Geometry check sheet. Reference: the model listing, model coordinates, mm. Give positions to 0.01 mm unless a question says otherwise; leave off trailing zeros. Order: outer loops, then holes, each group sorted by start corner. A loop starts at its lowest first (then second) coordinate and runs counter-clockwise, first axis right, second up. Notation, with made-up numbers: M 61.5,48.5 L 73.5,48.5 A10 cw 73.5,61.5 Z; hole C -32.5,-24.5 d10. An arc over 180 degrees is marked long. Answer as CSV lines item,"result". Start each with the question number.
Q1. Thickness scan on line 1 (Y direction, x = -12, z = -16.5); line 2 (Z direction, x = -14.25, y = 39.5); line 3 (Z direction, x = -20.25, y = 109). Record the ranges inside material, lowest first.
Q2. Go/stop test with flat-tipped pins: pin 1 (3.5 mm diameter, centred on x = -15.5, z = -15, fed in from -Y); pin 2 (2 mm diameter, centred on x = -14, y = 83, fed in from -Z); pin 3 (1 mm diameter, centred on y = 31.5, z = -14, fed in from -X). Record where each tip stops, or that it passes through.
Q3. Section check B-B, the plane y = 11.5. Record the boundary of the cut face in (x, z), then the cut area to 3 significant figures.
Q4. Section check A-A, the plane y = 162. Record the boundary of the cut face in (x, z), then the cut area to 3 significant figures.
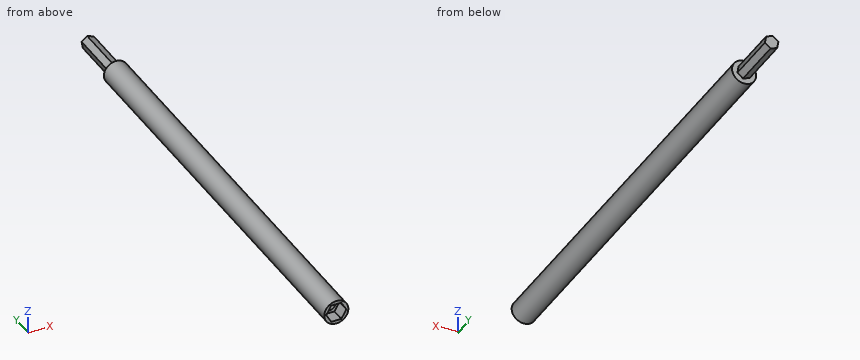
```python
from build123d import *

# Parameters (mm, degrees)
SKETCH1_R           = 4.5
SKETCH1_R_2         = 2.314285714
BOSS_EXTRUDE1_DEPTH = 160
SKETCH1_3_R         = 2.314285714
CUT_EXTRUDE1_DEPTH  = 5
BOSS_EXTRUDE2_DEPTH = 20


with BuildPart() as part:
    # Sketch1 → Boss-Extrude1 (new body)
    with BuildSketch(Plane(origin=(0, 0, 0), x_dir=(1, 0, 0), z_dir=(0, 1, 0))):
        with Locations((-16.157558946, 16.157558946)):
            Circle(SKETCH1_R)
        Polygon((-14.281170571, 12.907558946), (-12.404782196, 16.157558946), (-14.281170571, 19.407558946), (-18.033947321, 19.407558946), (-19.910335696, 16.157558946), (-18.033947321, 12.907558946), align=None, mode=Mode.SUBTRACT)
        Polygon((-18.033947321, 12.907558946), (-14.281170571, 12.907558946), (-12.404782196, 16.157558946), (-14.281170571, 19.407558946), (-18.033947321, 19.407558946), (-19.910335696, 16.157558946), align=None)
        with Locations((-16.157558946, 16.157558946)):
            Circle(SKETCH1_R_2, mode=Mode.SUBTRACT)
    extrude(amount=BOSS_EXTRUDE1_DEPTH)

    # Sketch1_3 → Cut-Extrude1 (cut)
    with BuildSketch(Plane(origin=(0, 0, 0), x_dir=(1, 0, 0), z_dir=(0, 1, 0))):
        Polygon((-18.033947321, 12.907558946), (-14.281170571, 12.907558946), (-12.404782196, 16.157558946), (-14.281170571, 19.407558946), (-18.033947321, 19.407558946), (-19.910335696, 16.157558946), align=None)
        with Locations((-16.157558946, 16.157558946)):
            Circle(SKETCH1_3_R, mode=Mode.SUBTRACT)
    extrude(amount=CUT_EXTRUDE1_DEPTH, mode=Mode.SUBTRACT)

    # Sketch2 → Boss-Extrude2 (add)
    with BuildSketch(Plane(origin=(0, 160, 0), x_dir=(1, 0, 0), z_dir=(0, 1, 0))):
        Polygon((-14.092245618, 14.462942882), (-13.657321721, 17.098864722), (-15.722635049, 18.793480786), (-18.222872273, 17.852175009), (-18.65779617, 15.216253169), (-16.592482843, 13.521637106), align=None)
    extrude(amount=BOSS_EXTRUDE2_DEPTH)


solid = part.part
```
Answer block:
1,line 1,"y = 0 to 160"
1,line 2,"z = -20.23 to -17.47, -14.85 to -12.08"
1,line 3,"z = -18.03 to -14.29"
2,pin 1,"stops at y = 5"
2,pin 2,"stops at z = -20.51"
2,pin 3,"stops at x = -20.34"
3,outline,"C -16.16,-16.16 d9; hole C -16.16,-16.16 d4.63"
3,area,"46.8 mm2"
4,outline,"M -18.66,-15.22 L -18.22,-17.85 L -15.72,-18.79 L -13.66,-17.1 L -14.09,-14.46 L -16.59,-13.52 Z"
4,area,"18.5 mm2"
